```python
from build123d import *

# Parameters (mm, degrees)
SKETCH1_R                            = 92.71
SKETCH1_R_2                          = 63.5
TOP_RING_DEPTH                       = 3.175
SKETCH2_R                            = 92.71
SKETCH2_R_2                          = 91.44
CYLINDRICAL_EXTENSTION_DEPTH         = 207.01
SKETCH3_R                            = 10.795
NOSE_CONE_EJECTION_CHARGE_HOLE_DEPTH = 210.185
SKETCH4_R                            = 5.08
CUT_EXTRUDE1_DEPTH                   = 3.175


with BuildPart() as part:
    # Sketch1 → Top Ring (new body)
    with BuildSketch(Plane(origin=(0, 0, 0), x_dir=(1, 0, 0), z_dir=(0, 1, 0))):
        Circle(SKETCH1_R)
        Circle(SKETCH1_R_2, mode=Mode.SUBTRACT)
    extrude(amount=TOP_RING_DEPTH)

    # Sketch2 → Cylindrical extenstion (add)
    with BuildSketch(Plane.XZ):
        Circle(SKETCH2_R)
        Circle(SKETCH2_R_2, mode=Mode.SUBTRACT)
    extrude(amount=CYLINDRICAL_EXTENSTION_DEPTH)

    # Sketch3 → Nose Cone Ejection Charge Hole (cut)
    with BuildSketch(Plane(origin=(0, 3.175, 0), x_dir=(1, 0, 0), z_dir=(0, 1, 0))):
        with Locations((81.223738514, -7.106156329)):
            Circle(SKETCH3_R)
    nose_cone_ejection_charge_hole = extrude(amount=-NOSE_CONE_EJECTION_CHARGE_HOLE_DEPTH, mode=Mode.SUBTRACT)

    # Nose Cone Ejection Charge Mirror: Nose Cone Ejection Charge Hole across plane
    add(nose_cone_ejection_charge_hole.mirror(Plane(origin=(0, 0, 0), x_dir=(0, 0, 1), z_dir=(1, 0, 0))), mode=Mode.SUBTRACT)

    # Sketch4 → Cut-Extrude1 (cut)
    with BuildSketch(Plane(origin=(0, 3.175, 0), x_dir=(1, 0, 0), z_dir=(0, 1, 0))):
        with Locations((53.881536726, -53.881536726)):
            Circle(SKETCH4_R)
        with Locations((-53.881536726, -53.881536726)):
            Circle(SKETCH4_R)
        with Locations((-53.881536726, 53.881536726)):
            Circle(SKETCH4_R)
        with Locations((53.881536726, 53.881536726)):
            Circle(SKETCH4_R)
    extrude(amount=-CUT_EXTRUDE1_DEPTH, mode=Mode.SUBTRACT)


solid = part.part
```
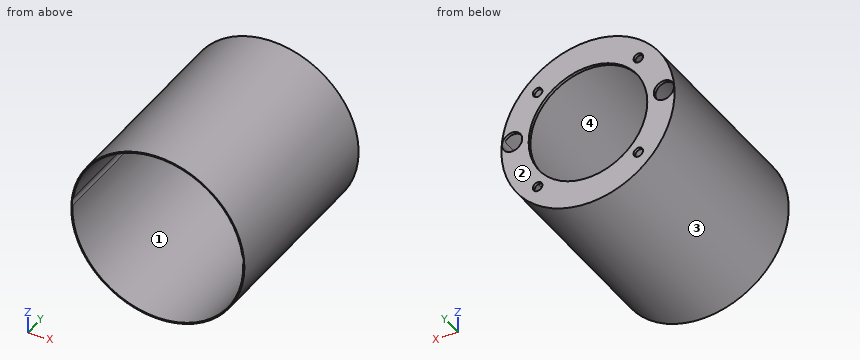
Check sheet for the modelled part. Datum: model origin and axes. Units: mm. Face numbers are marked on the shaded views. Give positions to 0.01 mm unless a question says otherwise; leave off trailing zeros. Write each loop counter-clockwise with the first axis right and the second up, starting at its lowest first coordinate (ties: lowest second). Pieces come first, ordered by that corner, then holes. Notation, with made-up numbers: (-35, 29) -> (20, 29) arc R19 cw to (20, 33) -> close; hole circle Ø6 at (81.25, 28). An arc over 180 degrees is marked (long way). Use CSV: the item, a comma, the result in double quotes. Start each with the question number.
Q1. Depth check by flat-ended pin: P1, Ø1.5, axis at x = -37, y = -98, coming from the -Z side; P2, Ø1.5, axis at x = -22.5, z = 70.5, coming from the -Y side; P3, Ø1.5, axis at y = -41, z = -69.5, coming from the -X side. Enter the tip coordinate at first touch or a pass-through.
Q2. Cross-section at B-B on y = -39. Enter the section's corners in (x, z) (3 decimals), and give its area (3 significant figures).
Q3. Release check for a two-part mould opening along X. For the marked faces 1, 2, 3 and 4 record: +X half, -X half, draft (parallel to the pull), parting line (faces both ways), or undercut.
Q4. Scan lines: line 1 along X through (y, z) = (-146.5, 2.5); line 2 along X through (y, z) = (-198, 11); line 3 along X through (y, z) = (1.7, 0). Record each from-to range of solid material in increasing order.
Working result:
1,P1,"stops at z = -85.33"
1,P2,"stops at y = 0"
1,P3,"stops at x = -62.2"
2,outline,"circle Ø185.42 at (0, 0); hole (-91.375, 3.435) arc R91.44 ccw (long way) to (91.375, 3.435) arc R10.795 ccw to (90.584, 12.484) arc R91.44 ccw to (-90.584, 12.484) arc R10.795 ccw to start"
2,area,"724 mm^2"
3,face 1,"undercut"
3,face 2,"draft"
3,face 3,"parting line"
3,face 4,"undercut"
4,line 1,"x = -92.68 to -91.41, 91.41 to 92.68"
4,line 2,"x = -92.06 to -91.29, 91.29 to 92.06"
4,line 3,"x = -92.71 to -89.35, -73.1 to -63.5, 63.5 to 73.1, 89.35 to 92.71"
